from build123d import *

# Parameters (mm, degrees)
BOSS_EXTRUDE1_DEPTH = 6.35
FILLET2_R           = 1.27
FILLET3_R           = 1.27


with BuildPart() as part:
    # Sketch1 → Boss-Extrude1 (new body)
    with BuildSketch(Plane.XY):
        Polygon((0, 0), (-101.6, 0), (0, 101.6), align=None)
    extrude(amount=BOSS_EXTRUDE1_DEPTH)

    # Fillet2
    fillet2_edges = [part.edges().sort_by_distance(p)[0] for p in [
        (-50.8, 50.8, 6.35),
    ]]
    fillet(fillet2_edges, radius=FILLET2_R)

    # Fillet3
    fillet3_edges = [part.edges().sort_by_distance(p)[0] for p in [
        (-50.8, 50.8, 0),
    ]]
    fillet(fillet3_edges, radius=FILLET3_R)


solid = part.part
For this review, take the finished solid that the model builds, in its own axes (mm). Give positions to 0.01 mm unless a question says otherwise; leave off trailing zeros. Order: outer loops, then holes, each group sorted by start corner. A loop starts at its lowest first (then second) coordinate and runs counter-clockwise, first axis right, second up. Notation, with made-up numbers: (3, 42) - (23, 42) arc R23 ccw to (23, 57) - close; hole circle Ø4 at (54.5, -6). An arc over 180 degrees is marked (long way). Answer as a JSON object with one key per item and string values. Group by question number.
Item 1: Clearance check with a flat-ended pin moving along its axis: pin 1 Ø3 at (x, z) = (-39.5, 5) entering from +Y. State where the tip first meets the part, or that it passes through.
Item 2: Take a section at A-A on z = 2.75. Give the boundary of the cut face in (x, y).
Item 3: Wall thickness on line 1 along Y through (x, z) = (-62.5, 2.75); line 2 along Y through (x, z) = (-42, 5.5); line 3 along X through (y, z) = (8, 4.5): over which ranges is each line inside the solid? List them lowest first.
Reported:
{
 "1": {"pin 1": "y = 63.6"},
 "2": {"outline": "(-101.6, 0) - (0, 0) - (0, 101.6) - close"},
 "3": {"line 1": "0 to 39.1", "line 2": "0 to 59.5", "line 3": "-93.6 to 0"}
}
